Read the model definition and answer for the solid it produces. Units are mm, in the model's axes. A direction names the side the tool comes from. Round coordinates to 2 decimals unless told otherwise and drop trailing zeros. Order: outer loops, then holes, each group sorted by start corner. A loop starts at its lowest first (then second) coordinate and runs counter-clockwise, first axis right, second up.
from build123d import *

# Parameters (mm, degrees)
SKETCH1_R                    = 7.5
BASE_FLANGE1_DEPTH           = 3.5
EDGE_FLANGE1_STRIP_W         = 21
EDGE_FLANGE1_STRIP_H         = 3.5
EDGE_FLANGE1_STRIP_CUT_DEPTH = 100
EDGE_FLANGE1_DEPTH           = 100
EDGE_FLANGE2_DEPTH           = 100
EDGE_FLANGE2_2_DEPTH         = 100
EDGE_FLANGE3_DEPTH           = 100
EDGE_FLANGE3_2_DEPTH         = 100
EDGE_FLANGE4_STRIP_W         = 21
EDGE_FLANGE4_STRIP_H         = 3.5
EDGE_FLANGE4_STRIP_CUT_DEPTH = 100
EDGE_FLANGE4_DEPTH           = 100
EDGE_FLANGE5_STRIP_W         = 21
EDGE_FLANGE5_STRIP_H         = 3.5
EDGE_FLANGE5_STRIP_CUT_DEPTH = 100
EDGE_FLANGE5_DEPTH           = 100
BREAK_CORNER1_START          = -0.79936489
BREAK_CORNER1_DEPTH          = 3.5
CUT_EXTRUDE1_DEPTH           = 10
CUT_EXTRUDE2_DEPTH           = 10


# Read off the part's stored shape, not the designer's step: Edge-Flange2, Edge-Flange3, Break-Corner1
# Sheet-metal steps are written as plain solids
with BuildPart() as part:
    # Sketch1 → Base-Flange1 (new body)
    with BuildSketch(Plane.XY):
        Polygon((90, 66), (100, 56), (100, 0), (0, 0), (0, 56), (10, 66), align=None)
        with Locations((19.875, 41)):
            Circle(SKETCH1_R, mode=Mode.SUBTRACT)
        with Locations((80.125, 41)):
            Circle(SKETCH1_R, mode=Mode.SUBTRACT)
    extrude(amount=-BASE_FLANGE1_DEPTH)

    # Edge-Flange1 strip (across the edge) → Edge-Flange1 strip cut (cut)
    with BuildSketch(Plane.YZ):
        with Locations((-3.5, -1.75)):
            Rectangle(EDGE_FLANGE1_STRIP_W, EDGE_FLANGE1_STRIP_H)
    extrude(amount=EDGE_FLANGE1_STRIP_CUT_DEPTH, mode=Mode.SUBTRACT)

    # Edge-Flange1 section (across the edge) → Edge-Flange1 (add)
    with BuildSketch(Plane.YZ):
        with BuildLine():
            Line((0, 3.5), (0, 61.5))
            Line((0, 61.5), (3.5, 61.5))
            Line((3.5, 61.5), (3.5, 3.5))
            ThreePointArc((3.5, 3.5), (4.525126266, 1.025126266), (7, 0))
            Line((7, 0), (7, -3.5))
            ThreePointArc((7, -3.5), (2.050252532, -1.449747468), (0, 3.5))
        make_face()
    extrude(amount=EDGE_FLANGE1_DEPTH)

    # Edge-Flange2 outline → Edge-Flange2 (cut)
    with BuildSketch(Plane.YZ):
        with BuildLine():
            ThreePointArc((0, 55.324651413), (0.937822174, 58.824651413), (3.5, 61.386829239))
            Line((3.5, 61.386829239), (3.5, 61.5))
            Line((3.5, 61.5), (0, 61.5))
            Line((0, 61.5), (0, 55.324651413))
        make_face()
    extrude(amount=EDGE_FLANGE2_DEPTH, mode=Mode.SUBTRACT)

    # Edge-Flange2 2 outline → Edge-Flange2 2 (add)
    with BuildSketch(Plane.YZ):
        with BuildLine():
            Line((59.20063511, 81.77337321), (4.605858997, 61.902499758))
            ThreePointArc((4.605858997, 61.902499758), (4.041672168, 61.668805922), (3.5, 61.386829239))
            Line((3.5, 61.386829239), (3.5, 55.324651413))
            ThreePointArc((3.5, 55.324651413), (4.132967845, 57.33216894), (5.802929498, 58.613575585))
            Line((5.802929498, 58.613575585), (60.397705611, 78.484449037))
            Line((60.397705611, 78.484449037), (59.20063511, 81.77337321))
        make_face()
    extrude(amount=EDGE_FLANGE2_2_DEPTH)

    # Edge-Flange3 outline → Edge-Flange3 (cut)
    with BuildSketch(Plane.YZ):
        with BuildLine():
            Line((59.20063511, 81.77337321), (59.094289381, 81.73466653))
            ThreePointArc((59.094289381, 81.73466653), (57.562946212, 78.450690506), (54.594776113, 76.372355428))
            Line((54.594776113, 76.372355428), (60.397705611, 78.484449037))
            Line((60.397705611, 78.484449037), (59.20063511, 81.77337321))
        make_face()
    extrude(amount=EDGE_FLANGE3_DEPTH, mode=Mode.SUBTRACT)

    # Edge-Flange3 2 outline → Edge-Flange3 2 (add)
    with BuildSketch(Plane.YZ):
        with BuildLine():
            ThreePointArc((59.094289381, 81.73466653), (59.173997997, 82.340113574), (59.20063511, 82.950203773))
            Line((59.20063511, 82.950203773), (59.20063511, 118.048751006))
            Line((59.20063511, 118.048751006), (55.70063511, 118.048751006))
            Line((55.70063511, 118.048751006), (55.70063511, 82.950203773))
            ThreePointArc((55.70063511, 82.950203773), (55.067667265, 80.942686246), (53.397705611, 79.661279601))
            Line((53.397705611, 79.661279601), (59.094289381, 81.73466653))
        make_face()
    extrude(amount=EDGE_FLANGE3_2_DEPTH)

    # Edge-Flange4 strip (across the edge) → Edge-Flange4 strip cut (cut)
    with BuildSketch(Plane(origin=(100, 55.70063511, 118.048751006), x_dir=(0, 0, -1), z_dir=(-1, 0, 0))):
        with Locations((-3.5, -1.75)):
            Rectangle(EDGE_FLANGE4_STRIP_W, EDGE_FLANGE4_STRIP_H)
    extrude(amount=EDGE_FLANGE4_STRIP_CUT_DEPTH, mode=Mode.SUBTRACT)

    # Edge-Flange4 section (across the edge) → Edge-Flange4 (add)
    with BuildSketch(Plane(origin=(100, 55.70063511, 118.048751006), x_dir=(0, 0, -1), z_dir=(-1, 0, 0))):
        with BuildLine():
            Line((0, 3.5), (0, 56.5))
            Line((0, 56.5), (3.5, 56.5))
            Line((3.5, 56.5), (3.5, 3.5))
            ThreePointArc((3.5, 3.5), (4.525126266, 1.025126266), (7, 0))
            Line((7, 0), (7, -3.5))
            ThreePointArc((7, -3.5), (2.050252532, -1.449747468), (0, 3.5))
        make_face()
    extrude(amount=EDGE_FLANGE4_DEPTH)

    # Edge-Flange5 strip (across the edge) → Edge-Flange5 strip cut (cut)
    with BuildSketch(Plane(origin=(100, -0.79936489, 114.548751006), x_dir=(0, 1, 0), z_dir=(-1, 0, 0))):
        with Locations((-3.5, -1.75)):
            Rectangle(EDGE_FLANGE5_STRIP_W, EDGE_FLANGE5_STRIP_H)
    extrude(amount=EDGE_FLANGE5_STRIP_CUT_DEPTH, mode=Mode.SUBTRACT)

    # Edge-Flange5 section (across the edge) → Edge-Flange5 (add)
    with BuildSketch(Plane(origin=(100, -0.79936489, 114.548751006), x_dir=(0, 1, 0), z_dir=(-1, 0, 0))):
        with BuildLine():
            Line((0, 3.5), (0, 21.5))
            Line((0, 21.5), (3.5, 21.5))
            Line((3.5, 21.5), (3.5, 3.5))
            ThreePointArc((3.5, 3.5), (4.525126266, 1.025126266), (7, 0))
            Line((7, 0), (7, -3.5))
            ThreePointArc((7, -3.5), (2.050252532, -1.449747468), (0, 3.5))
        make_face()
    extrude(amount=EDGE_FLANGE5_DEPTH)

    # Break-Corner1 outline → Break-Corner1 (cut)
    with BuildSketch(Plane(origin=(0, 0, 0), x_dir=(1, 0, 0), z_dir=(0, 1, 0)).offset(BREAK_CORNER1_START)):
        Polygon((100, -93.048751006), (90, -93.048751006), (100, -103.048751006), align=None)
        Polygon((0, -103.048751006), (10, -93.048751006), (0, -93.048751006), align=None)
    extrude(amount=BREAK_CORNER1_DEPTH, mode=Mode.SUBTRACT)

    # Sketch24 → Cut-Extrude1 (cut)
    with BuildSketch(Plane.XY.offset(118.048751006)):
        Polygon((70.663023535, 46.20063511), (80.663023535, 46.20063511), (92, 32.20063511), (82, 32.20063511), align=None)
        Polygon((38.663023535, 46.20063511), (48.663023535, 46.20063511), (60, 32.20063511), (50, 32.20063511), align=None)
        Polygon((6.663023535, 46.20063511), (16.663023535, 46.20063511), (28, 32.20063511), (18, 32.20063511), align=None)
        Polygon((18, 26.20063511), (6.663023535, 12.20063511), (16.663023535, 12.20063511), (28, 26.20063511), align=None)
        Polygon((50, 26.20063511), (38.663023535, 12.20063511), (48.663023535, 12.20063511), (60, 26.20063511), align=None)
        Polygon((82, 26.20063511), (70.663023535, 12.20063511), (80.663023535, 12.20063511), (92, 26.20063511), align=None)
    extrude(amount=-CUT_EXTRUDE1_DEPTH, mode=Mode.SUBTRACT)

    # Sketch25 → Cut-Extrude2 (cut)
    with BuildSketch(Plane(origin=(0, 3.5, 0), x_dir=(1, 0, 0), z_dir=(0, 1, 0))):
        with BuildLine():
            Line((41, -45.048751006), (41, -15.048751006))
            ThreePointArc((41, -15.048751006), (50, -6.048751006), (59, -15.048751006))
            Line((59, -15.048751006), (59, -45.048751006))
            ThreePointArc((59, -45.048751006), (50, -54.048751006), (41, -45.048751006))
        make_face()
    extrude(amount=-CUT_EXTRUDE2_DEPTH, mode=Mode.SUBTRACT)


solid = part.part
Q1. For a pull along Y with two mould halves and no side action, classify faces 5 (the face through (59, 2, 30)), 6 (the face through (22.25, 39.3, 116.32)), 7 (the face through (87, 32.201, 116)), 8 (the face through (95, 61, -2)) as released by +Y, released by -Y, zero draft, split by the parting line, or undercut.
Outcome:
face 5: zero draft
face 6: undercut
face 7: undercut
face 8: released by +Y
Q2. A cutting plane is placed at C-C, the plane y = 9. Give the vertices of the cut face in (x, z), plus the area to 3 significant figures.
Outcome:
outline: (0, -3.5) - (100, -3.5) - (100, 0) - (0, 0) - close; (0, 59.78) - (100, 59.78) - (100, 63.5) - (0, 63.5) - close; (0, 114.55) - (100, 114.55) - (100, 118.05) - (0, 118.05) - close
area: 1,070 mm2
Q3. Straight lines are drawn through the part: probe 1 along Z at (x, y) = (70.5, 11.5); probe 2 along Y at (x, z) = (16.5, 95.5); probe 3 along Z at (x, y) = (32.5, 19). For each, find the intervals that lie inside material, in ascending order.
Outcome:
probe 1: z = -3.5 to 0, 60.69 to 64.41, 114.55 to 118.05
probe 2: y = -0.8 to 2.7, 55.7 to 59.2
probe 3: z = -3.5 to 0, 63.42 to 67.14, 114.55 to 118.05
Q4. Flat-ended cylindrical pins translate along their axes: pin 1 (1.8 mm diameter, centred on x = 78, z = 116, fed in from -Y); pin 2 (1 mm diameter, centred on x = 77, z = 116.5, fed in from +Y); pin 3 (4 mm diameter, centred on x = 30.5, y = 1, fed in from -Z). Find the tip coordinate at first contact, or state that the pin passes through.
Outcome:
pin 1: stops at y = 0.49
pin 2: stops at y = 57.15
pin 3: stops at z = -2.24
Q5. A cutting plane is placed at B-B, the plane x = 36.5. Give the vertices of the cut face in (y, z), plus the area to 3 significant figures.
Outcome:
outline: (-0.8, 93.05) - (2.7, 93.05) - (2.7, 111.05) arc R3.5 cw to (6.2, 114.55) - (52.2, 114.55) arc R3.5 cw to (55.7, 111.05) - (55.7, 82.95) arc R3.5 cw to (53.4, 79.66) - (4.61, 61.9) arc R7 ccw to (0, 55.32) - (0, 3.5) arc R7 ccw to (7, -3.5) - (66, -3.5) - (66, 0) - (7, 0) arc R3.5 cw to (3.5, 3.5) - (3.5, 55.32) arc R3.5 cw to (5.8, 58.61) - (54.59, 76.37) arc R7 ccw to (59.2, 82.95) - (59.2, 111.05) arc R7 ccw to (52.2, 118.05) - (6.2, 118.05) arc R7 ccw to (-0.8, 111.05) - close
area: 1,020 mm2
Q6. A cutting plane is placed at A-A, the plane y = 41. Give the number of separate pieces and of enclosed holes in the cut face, plus the area to 3 significant figures.
Outcome:
separate pieces: 8
enclosed holes: 0
area: 862 mm2
Q7. A cutting plane is placed at D-D, the plane y = 23. Give the vertices of the cut face in (x, z), plus the area to 3 significant figures.
Outcome:
outline: (0, -3.5) - (100, -3.5) - (100, 0) - (0, 0) - close; (0, 64.87) - (100, 64.87) - (100, 68.6) - (0, 68.6) - close; (0, 114.55) - (15.41, 114.55) - (15.41, 118.05) - (0, 118.05) - close; (25.41, 114.55) - (47.41, 114.55) - (47.41, 118.05) - (25.41, 118.05) - close; (57.41, 114.55) - (79.41, 114.55) - (79.41, 118.05) - (57.41, 118.05) - close; (89.41, 114.55) - (100, 114.55) - (100, 118.05) - (89.41, 118.05) - close
area: 967 mm2
Q8. For faces 1 (the face through (49.8, 1.77, 6.05)), 2 (the face through (18.25, 33.68, -1.73)), 3 (the face through (54.25, 19.1, 116.32)), 4 (the face through (38, 3.5, 30)), determine the directions among +Z, -Z, +X, -X, +Y, -Y from which every point of the face is accessible in a straight line to the end or side of a thin tool.
Outcome:
face 1: +Y, -Y
face 2: -Z
face 3: +Z
face 4: +X, -X, +Y
